from build123d import *

# Parameters (mm, degrees)
SKETCH_W            = 35
SKETCH_H            = 6
PAD_DEPTH           = 2
SKETCH001_W         = 2
SKETCH001_H         = 1.75
SKETCH001_H_2       = 1
PAD001_DEPTH        = 9.5
SKETCH002_W         = 17
SKETCH002_H         = 6.5
SKETCH002_H_2       = 4
PAD002_DEPTH        = 2
SKETCH003_W         = 5
SKETCH003_H         = 1
SKETCH003_H_2       = 1.75
SKETCH003_H_3       = 2
PAD003_DEPTH        = 4.5
SKETCH004_W         = 88
SKETCH004_H         = 58
POCKET_DEPTH        = 2
SKETCH005_W         = 4
SKETCH005_H         = 0.8
PAD004_DEPTH        = 1
SKETCH006_W         = 4
SKETCH006_H         = 0.8
PAD005_DEPTH        = 1
PAD006_DEPTH        = 9.5
LINEARPATTERN_COUNT = 6
LINEARPATTERN_PITCH = 15
CHAMFER_SIZE        = 0.2


with BuildPart() as part:
    # Sketch → Pad (new body)
    with BuildSketch(Plane.XY):
        Polygon((-45, 30), (-45, 26.25), (-22, 26.25), (-22, 9.25), (-45, 9.25), (-45, 7.5), (-27, 7.5), (-27, -9.5), (-45, -9.5), (-45, -10.5), (-27, -10.5), (-27, -27.5), (-45, -27.5), (-45, -30), (45, -30), (45, 30), align=None)
        with Locations((18.89, -24.5)):
            Rectangle(SKETCH_W, SKETCH_H, mode=Mode.SUBTRACT)
    extrude(amount=PAD_DEPTH)

    # Sketch001 → Pad001 (new body)
    with BuildSketch(Plane.XY.offset(2)):
        with Locations((-44, 8.375)):
            Rectangle(SKETCH001_W, SKETCH001_H)
        with Locations((-44, -10)):
            Rectangle(SKETCH001_W, SKETCH001_H_2)
        Polygon((-45, -27.5), (-43, -27.5), (-43, -28.5), (43, -28.5), (43, 28.5), (-43, 28.5), (-43, 26.25), (-45, 26.25), (-45, 30), (45, 30), (45, -30), (-45, -30), align=None)
    extrude(amount=PAD001_DEPTH)

    # Sketch002 → Pad002 (new body)
    with BuildSketch(Plane(origin=(-45, 0, 0), x_dir=(0, -1, 0), z_dir=(-1, 0, 0))):
        with Locations((-17.75, 8.25)):
            Rectangle(SKETCH002_W, SKETCH002_H)
        with Locations((1, 9.5)):
            Rectangle(SKETCH002_W, SKETCH002_H_2)
        with Locations((19, 9.5)):
            Rectangle(SKETCH002_W, SKETCH002_H_2)
    extrude(amount=-PAD002_DEPTH)

    # Sketch003 → Pad003 (new body)
    with BuildSketch(Plane.XY.offset(2)):
        with Locations((-40.5, 28)):
            Rectangle(SKETCH003_W, SKETCH003_H)
        with Locations((-40.5, 8.375)):
            Rectangle(SKETCH003_W, SKETCH003_H_2)
        with Locations((-40.5, -10)):
            Rectangle(SKETCH003_W, SKETCH003_H)
        with Locations((-40.5, -28)):
            Rectangle(SKETCH003_W, SKETCH003_H)
        with Locations((40.5, -27.5)):
            Rectangle(SKETCH003_W, SKETCH003_H_3)
        with Locations((40.5, 27.5)):
            Rectangle(SKETCH003_W, SKETCH003_H_3)
    extrude(amount=PAD003_DEPTH)

    # Sketch004 → Pocket (cut)
    with BuildSketch(Plane.XY.offset(11.5)):
        Rectangle(SKETCH004_W, SKETCH004_H)
    extrude(amount=-POCKET_DEPTH, mode=Mode.SUBTRACT)

    # Sketch005 → Pad004 (new body)
    with BuildSketch(Plane.XZ.offset(-29)):
        with Locations((-30, 11.1)):
            Rectangle(SKETCH005_W, SKETCH005_H)
        with Locations((0, 11.1)):
            Rectangle(SKETCH005_W, SKETCH005_H)
        with Locations((30, 11.1)):
            Rectangle(SKETCH005_W, SKETCH005_H)
    extrude(amount=PAD004_DEPTH)

    # Sketch006 → Pad005 (new body)
    with BuildSketch(Plane(origin=(0, -29, 0), x_dir=(-1, 0, 0), z_dir=(0, 1, 0))):
        with Locations((-30, 11.1)):
            Rectangle(SKETCH006_W, SKETCH006_H)
        with Locations((0, 11.1)):
            Rectangle(SKETCH006_W, SKETCH006_H)
        with Locations((30, 11.1)):
            Rectangle(SKETCH006_W, SKETCH006_H)
    extrude(amount=PAD005_DEPTH)

    # Sketch007 → Pad006 (new body)
    with BuildSketch(Plane(origin=(0, 0, 0), x_dir=(1, 0, 0), z_dir=(0, 0, -1))):
        with BuildLine():
            Line((36.25, 31), (36.25, 30))
            Line((36.25, 30), (38.75, 30))
            Line((38.75, 30), (38.75, 31))
            ThreePointArc((38.75, 31), (39.396907, 31.696052), (39.689917, 32.6))
            Line((38.689917, 32.6), (39.689917, 32.6))
            Line((37.5, 30.810387), (38.689917, 32.6))
            Line((36.310083, 32.6), (37.5, 30.810387))
            Line((35.310083, 32.6), (36.310083, 32.6))
            ThreePointArc((35.310083, 32.6), (35.603093, 31.696052), (36.25, 31))
        make_face()
        with BuildLine():
            Line((36.25, -30), (36.25, -31))
            ThreePointArc((36.25, -31), (35.603093, -31.696052), (35.310083, -32.6))
            Line((35.310083, -32.6), (36.310083, -32.6))
            Line((37.5, -30.6), (36.310083, -32.6))
            Line((38.689917, -32.6), (37.5, -30.6))
            Line((39.689917, -32.6), (38.689917, -32.6))
            ThreePointArc((39.689917, -32.6), (39.396907, -31.696052), (38.75, -31))
            Line((38.75, -30), (38.75, -31))
            Line((36.25, -30), (38.75, -30))
        make_face()
    pad006 = extrude(amount=-PAD006_DEPTH)

    # LinearPattern: Pad006 ×6
    with Locations(*[(-i * LINEARPATTERN_PITCH, 0, 0) for i in range(1, LINEARPATTERN_COUNT)]):
        add(pad006)

    # Chamfer
    chamfer_edges = [part.edges().sort_by_distance(p)[0] for p in [
        (0, 28, 11.5),
        (-30, 28, 11.5),
        (30, 28, 11.5),
        (-30, -28, 11.5),
        (0, -28, 11.5),
        (30, -28, 11.5),
    ]]
    chamfer(chamfer_edges, length=CHAMFER_SIZE)


solid = part.part
The listing builds one solid part. Answer for the finished solid, in the listing's coordinates (mm). A direction names the side the tool comes from. Give positions to 0.01 mm unless a question says otherwise; leave off trailing zeros. Loops run counter-clockwise (first coordinate to the right, second up) from the corner with the lowest first, then second, coordinate; pieces in that order, holes last. Notation, with made-up numbers: (43, 35.5) - (73, 35.5) arc R16 ccw to (73, 50.5) - close; hole circle Ø10 at (-23.5, -10). An arc over 180 degrees is marked (long way). Use one line per item in the form item = value.
1. Which of the six approach directions +Z, -Z, +X, -X, +Y, -Y give full straight-line access (tool end or side, diameter ignored) to faces 4 (the face through (-40, -9.5, 3)), 5 (the face through (36.39, -25, 1)), 6 (the face through (40, -27, 6.5)), 7 (the face through (-27, -1, 1)), 8 (the face through (37, 31, 9.5))?
Calculated:
face_4 = -Z, -X
face_5 = +Z, -Z
face_6 = +Z
face_7 = +Z, -Z, -X
face_8 = +Z, +X, -X, +Y
2. The mould has two halves that part along X. Classify faces 1 (the face through (7, -31, 9.5)), 2 (the face through (-23.103, -31.718, 4.684)), 3 (the face through (-27, -19, 1)): pulls with the +X half, pulls with the -X half, needs draft (parallel to the pull), parting line crosses it, or undercut.
Calculated:
face_1 = needs draft
face_2 = undercut
face_3 = pulls with the -X half
3. Find the intervals of material crossed by line 1 along Y through (x, z) = (0, 11.25); line 2 along X through (y, z) = (26, 11.25); line 3 along Y through (x, z) = (-19, 6.25), in increasing order. Write a range as [from, to].
Calculated:
line_1 = [-30, -28], [28, 30]
line_2 = [-45, -44], [44, 45]
line_3 = [-30, -28.5], [28.5, 30]
4. Given pin 1 Ø5 at (x, z) = (17.5, 3) entering from +Y; pin 2 Ø8 at (x, y) = (-15.5, 1) entering from -Z; pin 3 Ø10 at (x, y) = (-25.5, -12.5) entering from +Z; pin 4 Ø0.8 at (y, z) = (30.5, 3.5) entering from -X, each flat-ended and moving along its own axis, determine where each tip first touches the part or whether it passes through.
Calculated:
pin_1 = 30
pin_2 = 0
pin_3 = 2
pin_4 = -38.75
5. Section A-A on x = 31 is taken. Give the vertices of the cut face in (y, z), then the cut area to 3 significant figures.
Calculated:
outline = (-30, 0) - (-27.5, 0) - (-27.5, 2) - (-28.5, 2) - (-28.5, 9.5) - (-29, 9.5) - (-29, 10.7) - (-28, 10.7) - (-28, 11.3) - (-28.2, 11.5) - (-30, 11.5) - close; (-21.5, 0) - (30, 0) - (30, 11.5) - (28.2, 11.5) - (28, 11.3) - (28, 10.7) - (29, 10.7) - (29, 9.5) - (28.5, 9.5) - (28.5, 2) - (-21.5, 2) - close
area = 136 mm^2
6. Section B-B on x = -34 is taken. Give the vertices of the cut face in (y, z).
Calculated:
outline = (-30, 0) - (-27.5, 0) - (-27.5, 2) - (-28.5, 2) - (-28.5, 9.5) - (-29, 9.5) - (-29, 11.5) - (-30, 11.5) - close; (-10.5, 0) - (-9.5, 0) - (-9.5, 2) - (-10.5, 2) - close; (7.5, 0) - (9.25, 0) - (9.25, 2) - (7.5, 2) - close; (26.25, 0) - (30, 0) - (30, 11.5) - (29, 11.5) - (29, 9.5) - (28.5, 9.5) - (28.5, 2) - (26.25, 2) - close
7. Section D-D on y = 19 is taken. Give the vertices of the cut face in (x, z).
Calculated:
outline = (-45, 5) - (-43, 5) - (-43, 9.5) - (-44, 9.5) - (-44, 11.5) - (-45, 11.5) - close; (-22, 0) - (45, 0) - (45, 11.5) - (44, 11.5) - (44, 9.5) - (43, 9.5) - (43, 2) - (-22, 2) - close
8. Section C-C on y = 5.5 is taken. Give the vertices of the cut face in (x, z), then the cut area to 3 significant figures.
Calculated:
outline = (-45, 7.5) - (-43, 7.5) - (-43, 9.5) - (-44, 9.5) - (-44, 11.5) - (-45, 11.5) - close; (-27, 0) - (45, 0) - (45, 11.5) - (44, 11.5) - (44, 9.5) - (43, 9.5) - (43, 2) - (-27, 2) - close
area = 167 mm^2
